Geometry check sheet. Reference: the model listing, model coordinates, mm. Round coordinates to 2 decimals unless told otherwise and drop trailing zeros. Order: outer loops, then holes, each group sorted by start corner. A loop starts at its lowest first (then second) coordinate and runs counter-clockwise, first axis right, second up.
(1) Sectioned sample at B-B (z = 22.5). Record the boundary of the cut face in (x, y).
(2) Sectioned sample at A-A (y = -4.5). Record the boundary of the cut face in (x, z).
(3) Material ranges on line 1 along Y through (x, z) = (7.75, 19); line 2 along Z through (x, y) = (9, -43); line 3 along X through (y, z) = (-47, 19.5), recorded low to high.
(4) Sectioned sample at D-D (x = 22.25). Record the boundary of the cut face in (y, z).
(5) Sectioned sample at C-C (x = 13). Record the boundary of the cut face in (y, z), plus the area to 3 significant figures.
(6) Go/stop test with flat-tipped pins: pin 1 (3.5 mm diameter, centred on y = -76, z = 4, fed in from -X); pin 2 (3 mm diameter, centred on y = 2.5, z = 21.5, fed in from +X); pin 3 (6 mm diameter, centred on y = -53.5, z = 9, fed in from +X). Record where each tip stops, or that it passes through.
from build123d import *

# Parameters (mm, degrees)
F0_W     = 10.16
F0_H     = 3.3
F0_W_2   = 3.3
F0_H_2   = 10.16
F1_DEPTH = 73.4
F2_DEPTH = 3.5
F4_W     = 3.3
F4_H     = 10.16
F4_W_2   = 10.16
F4_H_2   = 3.3
F5_DEPTH = 3.5
F7_DEPTH = 73.4


with BuildPart() as f1:
    # F0 (on Front) → F1 (new body)
    with BuildSketch(Plane.XZ):
        with BuildLine():
            Line((0, 50), (0, 0))
            Line((0, 0), (30, 0))
            ThreePointArc((30, 0), (8.0754008763, 20.8452405258), (0, 50))
        make_face()
        with Locations((11.08, 4.19)):
            Rectangle(F0_W, F0_H, mode=Mode.SUBTRACT)
        with Locations((2.92, 19.7566125902)):
            Rectangle(F0_W_2, F0_H_2, mode=Mode.SUBTRACT)
        with Locations((2.92, 19.7566125902)):
            Rectangle(F0_W_2, F0_H_2)
        with Locations((11.08, 4.19)):
            Rectangle(F0_W, F0_H)
    extrude(amount=F1_DEPTH)

    # F0 (on Front) → F2 (join)
    with BuildSketch(Plane.XZ):
        with Locations((2.92, 19.7566125902)):
            Rectangle(F0_W_2, F0_H_2)
        with Locations((11.08, 4.19)):
            Rectangle(F0_W, F0_H)
    extrude(amount=-F2_DEPTH)

    # F4 (on offset) → F5 (join)
    with BuildSketch(Plane.XZ.offset(73.4)):
        with Locations((2.92, 20.32)):
            Rectangle(F4_W, F4_H)
        with Locations((11.08, 4.19)):
            Rectangle(F4_W_2, F4_H_2)
    extrude(amount=F5_DEPTH)

    # F6 (on offset) → F7 (join)
    with BuildSketch(Plane.XZ.offset(73.4)):
        with BuildLine():
            ThreePointArc((8.0754008763, 20.8452405258), (9.5386255261, 18.5347993911), (11.1116185287, 16.297645479))
            Line((11.1116185287, 16.297645479), (11.1116185287, 20.8452405258))
            Line((11.1116185287, 20.8452405258), (10.6401696458, 20.8452405258))
            Line((10.6401696458, 20.8452405258), (8.0754008763, 20.8452405258))
        make_face()
    extrude(amount=-F7_DEPTH)


solid = f1.part
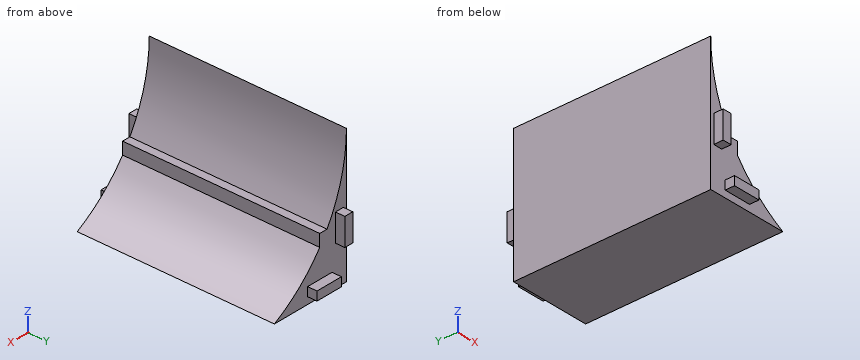
Answer below:
1. outline: (0, -73.4) - (1.27, -73.4) - (1.27, -76.9) - (4.57, -76.9) - (4.57, -73.4) - (7.12, -73.4) - (7.12, 0) - (4.57, 0) - (4.57, 3.5) - (1.27, 3.5) - (1.27, 0) - (0, 0) - close
2. outline: (0, 0) - (30, 0) arc R56.67 cw to (11.11, 16.3) - (11.11, 20.85) - (8.08, 20.85) arc R56.67 cw to (0, 50) - close
3. line 1: y = -73.4 to 0
3. line 2: z = 0 to 20.85
3. line 3: x = 0 to 11.11
4. outline: (-73.4, 0) - (0, 0) - (0, 4.98) - (-73.4, 4.98) - close
5. outline: (-76.9, 2.54) - (-73.4, 2.54) - (-73.4, 0) - (0, 0) - (0, 2.54) - (3.5, 2.54) - (3.5, 5.84) - (0, 5.84) - (0, 13.88) - (-73.4, 13.88) - (-73.4, 5.84) - (-76.9, 5.84) - close
5. area: 1,040 mm2
6. pin 1: stops at x = 6
6. pin 2: stops at x = 4.57
6. pin 3: stops at x = 20.96
